Verification items for the finished model (mm, model axes). A direction names the side the tool comes from. Coordinates: 2 decimals unless noted, no trailing zeros. Loops run counter-clockwise (first coordinate to the right, second up) from the corner with the lowest first, then second, coordinate; pieces in that order, holes last. Notation, with made-up numbers: (31, 17.5) - (60, 17.5) arc R12 ccw to (60, 35.5) - close; hole circle Ø6 at (48.25, -1.5). An arc over 180 degrees is marked (long way). Answer as CSV lines item,"result". Start each with the question number.
1. Cross-section at A-A (x = 26). Enter the section's corners in (y, z) (3 decimals), plus the area to 3 significant figures.
2. Set-up check for faces 1 (the flat face through (20, 8, -20)), 2 (the flat face through (-6, 100, -14)), 3 (the flat face through (-8.232, 104.542, -14.16)), 4 (the flat face through (15, 46, -30)), 5 (the flat face through (22.1, 21.5, -13)): record each of +Z, -Z, +X, -X, +Y, -Y from which the full face is reachable in a straight line by a thin tool's end or side.
3. Cross-section at C-C (z = -15). State how many separate pieces and enclosed holes the cut face has, plus the area to 3 significant figures.
4. Cross-section at D-D (z = -66.5). Enter the section's corners in (x, y), plus the area to 3 significant figures.
5. Gauge pin test, flat ends, axial feed: P1, Ø15, axis at x = 20, z = -61.5, coming from the -Y side; P2, Ø1.5, axis at y = 100.5, z = -5.5, coming from the +X side; P3, Ø8, axis at x = 2.5, y = 65.5, coming from the -Z side; P4, Ø16, axis at x = 9.5, z = -13, coming from the -Y side. Record the tip position at first contact, or that the pin passes through.
6. Material ranges on line 1 (Y direction, x = 26.5, z = -15) (3 decimals); line 2 (Y direction, x = 28.25, z = -15) (3 decimals); line 3 (Z direction, x = 25, y = 15), recorded low to high. Write a range as [from, to].
7. Cross-section at B-B (y = 15.06). Enter the section's corners in (x, z) (3 decimals), plus the area to 4 significant figures.
Autodesk Inventor part; units mm, degrees
ref_plane "Work Plane1" through (0, 0, -15) normal (0, 0, 1) x (1, 0, 0)
ref_plane "YZ Plane" through (0, 0, 0) normal (1, 0, 0) x (0, 1, 0)
ref_plane "XZ Plane" through (0, 0, 0) normal (0, 1, 0) x (-1, 0, 0)
sketch "Sketch1" plane through (0, 0, 0) normal (0, 0, 1) x (1, 0, 0)
  line L0 (0, 0) -> (25, 0)
  line L1 (25, 0) -> (25, 40)
  line L2 (25, 40) -> (0, 40)
  line L3 (0, 40) -> (0, 0)
  dimension "d1" = 25
  dimension "d2" = 40
  dimension "d3" = 25
extrude "Extrusion1" add sketch "Sketch1" against normal blind 30
sketch "Sketch2" plane through (25, 0, 0) normal (1, 0, 0) x (0, 0, -1)
  line L0 (0, 0) -> (30, 0)
  circle A0 centre (15, 6.56) radius 2.46
extrude "Extrusion2" cut sketch "Sketch2" against normal blind 30
sketch "Sketch3" plane through (0, 0, 0) normal (-1, 0, 0) x (0, 0, 1)
  line L0 (0, 0) -> (-30, 0)
  line L1 (-25.05, 0) -> (-4.95, 0)
  line L2 (-4.95, 0) -> (-4.95, 33.12)
  line L3 (-4.95, 33.12) -> (-25.05, 33.12)
  line L4 (-25.05, 33.12) -> (-25.05, 0)
  dimension "d11" = 20.1
extrude "Extrusion3" cut sketch "Sketch3" against normal blind 20
sketch "Sketch4" plane through (0, 0, 0) normal (0, -1, 0) x (1, 0, 0)
  line L0 (20, -4.95) -> (20, -25.05)
  line L1 (20, -15) -> (25, -15)
  line L2 (25, 0) -> (25, -30)
  line L3 (20, -8.025) -> (25, -8.025)
  line L4 (25, -8.025) -> (25, -21.975)
  line L5 (25, -21.975) -> (20, -21.975)
  line L6 (20, -21.975) -> (20, -8.025)
  line L7 (20, -8.025) -> (25, -21.975) construction
  line L8 (25, -8.025) -> (20, -21.975) construction
  line L9 (25, -12.54) -> (25, -17.46)
  point P0 (0, 0)
  point P1 (22.5, -15)
  dimension "d14" = 13.95
extrude "Extrusion4" add sketch "Sketch4" along normal blind 15
sketch "Sketch5" plane through (20, 0, 0) normal (-1, 0, 0) x (0, 0, 1)
  circle A0 centre (-15, 6.56) radius 2.46
  circle A1 centre (-15, 6.56) radius 4.7025
  circle A2 centre (-15, 6.56) radius 2.46
  circle A3 centre (-15, 6.56) radius 2.46
  point P0 (0, 0)
  dimension "d17" = 9.405
extrude "Extrusion5" cut sketch "Sketch5" against normal blind 2.1
sketch "Sketch6" plane through (25, 0, 0) normal (1, 0, 0) x (0, 0, -1)
  circle A0 centre (15, 6.56) radius 4.7025
  line L0 (15, 6.56) -> (15, 23.56)
  circle A1 centre (15, 23.56) radius 2.46
  point P0 (0, 0)
  dimension "d20" = 17
  dimension "d21" = 4.92
extrude "Extrusion6" cut sketch "Sketch6" against normal blind 10 contours A1
sketch "Sketch7" plane through (20, 0, 0) normal (-1, 0, 0) x (0, 0, 1)
  circle A0 centre (-15, 23.56) radius 2.46
  circle A1 centre (-15, 23.56) radius 4.7025
  point P0 (0, 0)
  dimension "d24" = 9.405
extrude "Extrusion7" cut sketch "Sketch7" against normal blind 2.1
sketch "Sketch9" plane through (25, 0, 0) normal (1, 0, 0) x (0, 0, -1)
  circle A0 centre (15, 6.56) radius 2.46
  circle A1 centre (15, 6.56) radius 2.46
  circle A2 centre (15, 23.56) radius 2.46
  circle A3 centre (15, 23.56) radius 2.46
  line L0 (30, 40) -> (30, 0)
  line L1 (30, 0) -> (30, 40)
  line L2 (30, 40) -> (0, 40)
  line L3 (0, 40) -> (0, 0)
  line L4 (0, 0) -> (8.025, 0)
  line L5 (21.975, 0) -> (21.975, -15)
  line L6 (21.975, -15) -> (8.025, -15)
  line L7 (8.025, -15) -> (8.025, 0)
  line L8 (0, 0) -> (8.025, 0)
  line L9 (21.975, 0) -> (30, 0)
extrude "Extrusion8" add sketch "Sketch9" along normal blind 5
sketch "Sketch10" plane through (0, 40, 0) normal (0, 1, 0) x (1, 0, 0)
  line L0 (0, 30) -> (30, 30)
  line L1 (30, 0) -> (0, 0)
  line L2 (0, 30) -> (30, 30)
  line L3 (30, 30) -> (30, 0)
  line L4 (30, 0) -> (0, 0)
  line L5 (0, 0) -> (0, 30)
extrude "Extrusion9" add sketch "Sketch10" along normal blind 30
sketch "Sketch12" plane through (30, 0, 0) normal (1, 0, 0) x (0, 0, -1)
  circle A0 centre (15, 6.56) radius 2.46
  line L0 (15, 6.56) -> (15, 15.06)
  circle A1 centre (15, 15.06) radius 2.525
  point P0 (0, 0)
  dimension "d31" = 8.5
  dimension "d33" = 5.05
extrude "Extrusion10" cut sketch "Sketch12" against normal blind 30 contours A1
sketch "Sketch14" plane through (0, 0, 0) normal (0, 0, 1) x (1, 0, 0)
  line L0 (30, 70) -> (0, 70)
  line L1 (0, 70) -> (0, 85)
  line L2 (30, 100) -> (15, 115)
  line L3 (-12, 115) -> (15, 115)
  line L4 (30, 0) -> (30, 70)
  line L5 (30, 100) -> (30, 70)
  line L6 (-9.5, 113.5) -> (-12, 115)
  line L7 (-9.5, 101.5) -> (-12, 100)
  line L8 (-7, 107.5) -> (-9.5, 101.5)
  line L9 (-7, 107.5) -> (-9.5, 113.5)
  line L10 (0, 100) -> (0, 85)
  line L11 (0, 100) -> (-12, 100)
  point P0 (0, 0)
  dimension "d49" = 15
  dimension "d61" = 12
extrude "Extrusion12" add sketch "Sketch14" against normal blind 30
sketch "Sketch15" plane through (0, 0, -25.05) normal (-1, 0, 0) x (0, 0, 1)
  line L0 (0, 33.12) -> (20.1, 33.12)
  line L1 (20.1, 33.12) -> (20.1, 0)
  line L2 (0, 33.12) -> (20.1, 33.12)
  line L3 (20.1, 33.12) -> (20.1, 31.1)
  line L4 (20.1, 31.1) -> (0, 31.1)
  line L5 (0, 31.1) -> (0, 33.12)
  point P0 (25.05, 0)
  dimension "d57" = 2.02
extrude "Extrusion13" add sketch "Sketch15" against normal blind 20
sketch "Sketch19" plane through (0, 0, 0) normal (0, 0, 1) x (1, 0, 0)
  line L0 (0, 100) -> (0, 0)
  line L1 (0, 100) -> (-12, 100)
  line L2 (0, 100) -> (-12, 100)
  line L3 (-12, 100) -> (-9.5, 101.5)
  line L4 (-12, 100) -> (-9.5, 101.5)
  line L5 (-9.5, 101.5) -> (-7, 107.5)
  line L6 (-9.5, 101.5) -> (-7, 107.5)
  line L7 (-7, 107.5) -> (-9.5, 113.5)
  line L8 (-7, 107.5) -> (-9.5, 113.5)
  line L9 (-9.5, 113.5) -> (-12, 115)
  line L10 (-9.5, 113.5) -> (-12, 115)
  line L11 (-12, 115) -> (15, 115)
  line L12 (-12, 115) -> (15, 115)
  line L13 (15, 115) -> (30, 100)
  line L14 (15, 115) -> (30, 100)
  line L15 (30, 100) -> (30, 90)
  line L16 (30, 0) -> (30, 100)
  line L17 (30, 90) -> (0, 90)
  line L18 (0, 0) -> (0, 100)
  line L19 (0, 90) -> (0, 100)
  dimension "d62" = 10
  dimension "d63" = 30
extrude "Extrusion14" add sketch "Sketch19" along normal blind 45
ref_plane "Work Plane1" through (0, 0, -15) normal (0, 0, 1) x (1, 0, 0)
mirror "Mirror1" about plane through (0, 0, -15) normal (0, 0, 1) of "Extrusion14"
properties part number "rec_b_12mm_x_120mm"
Values follow:
1,outline,"(-15, -21.975) - (0, -21.975) - (0, -30) - (90, -30) - (90, -75) - (104, -75) - (104, 45) - (90, 45) - (90, 0) - (0, 0) - (0, -8.025) - (-15, -8.025) - close; hole circle Ø4.92 at (6.56, -15); hole circle Ø5.05 at (15.06, -15); hole circle Ø4.92 at (23.56, -15)"
1,area,"4,530 mm²"
2,face 1,"-X, -Y"
2,face 2,"+Z, -Z, -X, -Y"
2,face 3,"+Z, -Z, -X"
2,face 4,"-Z, +X, -X, -Y"
2,face 5,"-X"
3,separate pieces,"4"
3,enclosed holes,"0"
3,area,"2,830 mm²"
4,outline,"(-12, 100) - (0, 100) - (0, 90) - (30, 90) - (30, 100) - (15, 115) - (-12, 115) - (-9.5, 113.5) - (-7, 107.5) - (-9.5, 101.5) - close"
4,area,"769 mm²"
5,P1,"stops at y = 90"
5,P2,"stops at x = 30"
5,P3,"stops at z = -30"
5,P4,"stops at y = 31.1"
6,line 1,"y = [-15, 4.1], [9.02, 12.535], [17.585, 21.1], [26.02, 103.5]"
6,line 2,"y = [-15, 4.1], [9.02, 12.535], [17.585, 21.1], [26.02, 101.75]"
6,line 3,"z = [-30, -17.52], [-12.48, 0]"
7,outline,"(0, -30) - (30, -30) - (30, -17.525) - (20, -17.525) - (20, -25.05) - (0, -25.05) - close; (0, -4.95) - (20, -4.95) - (20, -12.475) - (30, -12.475) - (30, 0) - (0, 0) - close"
7,area,"447.5 mm²"
